Here's how the part is built. I have some questions about the finished solid (model axes, mm). Coordinates: 2 decimals unless noted, no trailing zeros. Order: outer loops, then holes, each group sorted by start corner. A loop starts at its lowest first (then second) coordinate and runs counter-clockwise, first axis right, second up. Notation, with made-up numbers: (-19.5, 53.25) - (-14.5, 53.25) arc R28 cw to (-14.5, 71.25) - close; hole circle Ø1 at (74, -0.75). An arc over 180 degrees is marked (long way). Use CSV: the item, a comma, the result in double quotes. Start each with the question number.
from build123d import *

# Parameters (mm, degrees)
F0_W     = 101.6
F0_H     = 609.6
F0_R     = 14.921552
F1_DEPTH = 12.7
F2_DEPTH = 12.7


with BuildPart() as f1:
    # F0 (on Right) → F1 (new body)
    with BuildSketch(Plane.YZ):
        with Locations((-5.578191, -6.483793)):
            Rectangle(F0_W, F0_H)
        with Locations((-5.578191, -108.083793)):
            Circle(F0_R, mode=Mode.SUBTRACT)
    extrude(amount=F1_DEPTH)

    # F0 (on Right) → F2 (join)
    with BuildSketch(Plane.YZ):
        with Locations((-5.578191, -6.483793)):
            Rectangle(F0_W, F0_H)
        with Locations((-5.578191, -108.083793)):
            Circle(F0_R, mode=Mode.SUBTRACT)
    extrude(amount=F2_DEPTH)


solid = f1.part
Item 1: Suppose I cut it at A-A on z = -100. Write out the boundary of the cut face in (x, y).
Item 2: Suppose I cut it at B-B on y = 0. Write out the boundary of the cut face in (x, z).
Item 3: We'd pull the mould along Z, two halves only. Please class faces 1 (the flat face through (0, -6, -2)), 2 (the flat face through (6, -6, -311.284)), 3 (the cylindrical face through (6.26, -8.81, -122.65)): released by +Z, released by -Z, zero draft, split by the parting line, or undercut.
Item 4: Please list where this line runs through material, in increasing order: line 1 along Z through (x, y) = (3, 7). Write a range as from..to.
Item 5: For pin 1 Ø4 at (y, z) = (32, -227.5) entering from -X, with a flat end and sliding along its axis, tell me the tip position at first contact or that it passes through.
Here are the results:
1,outline,"(0, -56.38) - (12.7, -56.38) - (12.7, -18.12) - (0, -18.12) - close; (0, 6.96) - (12.7, 6.96) - (12.7, 45.22) - (0, 45.22) - close"
2,outline,"(0, -311.28) - (12.7, -311.28) - (12.7, -121.92) - (0, -121.92) - close; (0, -94.24) - (12.7, -94.24) - (12.7, 298.32) - (0, 298.32) - close"
3,face 1,"zero draft"
3,face 2,"released by -Z"
3,face 3,"undercut"
4,line 1,"-311.28..-116.11, -100.06..298.32"
5,pin 1,"x = 0"
